Job drawing, mm, ordinate dimensions from the low corner. One solid piece. A direction names the side the tool comes from. Give positions to 0.01 mm unless a question says otherwise; leave off trailing zeros. Order: outer loops, then holes, each group sorted by start corner. A loop starts at its lowest first (then second) coordinate and runs counter-clockwise, first axis right, second up. Notation, with made-up numbers: M 52,7 L 86,7 A14 cw 86,33 Z; hole C 24,-38.5 d1. An arc over 180 degrees is marked long. Use CSV: the item, a comma, the result in double quotes. Start each with the question number.
Item 1: Pin check, flat tips, straight feed: P1, Ø23, axis at x = 42, y = 43.5, coming from the +Z side; P2, Ø7.5, axis at x = 54, y = 95, coming from the +Z side; P3, Ø12.5, axis at x = 50.5, z = 11.5, coming from the -Y side. Stop position of each tip, or through.
Item 2: Band-saw the part on C-C on x = 80.5. Write the cut outline in (y, z).
Item 3: Which spindle directions (+Z, -Z, +X, -X, +Y, -Y) get a long thin tool onto all of the face, cutting with end or side? Do the marked faces 5, 6, 7 and 8. Say none if no direction does.
Item 4: Two-plate mould, pull along X, no slides. Class the marked faces 1, 2, 3 and 4: pulls with the +X half, pulls with the -X half, needs draft (parallel to the pull), parting line crosses it, or undercut.
Item 5: Band-saw the part on A-A on y = 12.5. Write the cut outline in (x, z), plus the area to 3 significant figures.
Item 6: Band-saw the part on D-D on z = 13. Write the cut outline in (x, y), plus the area to 3 significant figures.
Item 7: Band-saw the part on B-B on z = 62. Write the cut outline in (x, y).
Item 8: Wall check: line 1 along X through (y, z) = (93, 73); line 2 along Z through (x, y) = (4, 30); line 3 along Y through (x, z) = (86, 84.5). Give the ranges that are in metal, low to high.
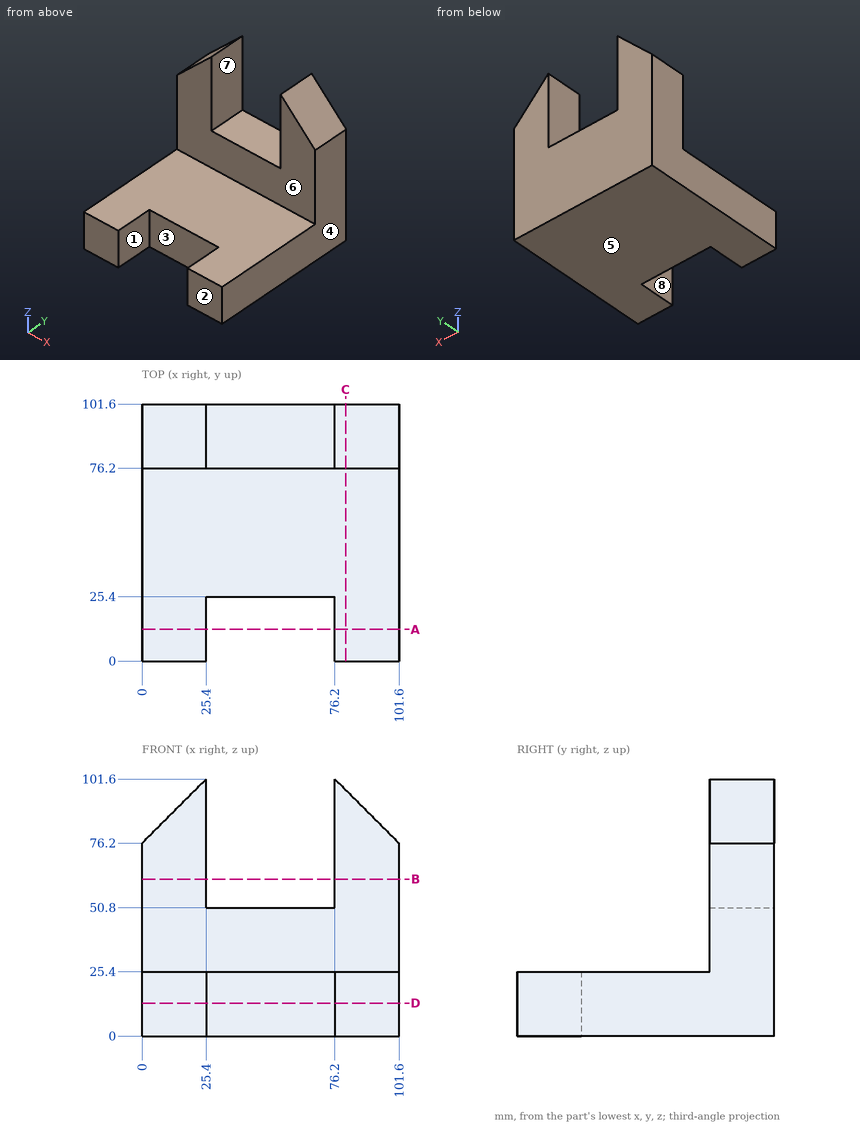
Model answer:
1,P1,"stops at z = 25.4"
1,P2,"stops at z = 50.8"
1,P3,"stops at y = 25.4"
2,outline,"M 0,0 L 101.6,0 L 101.6,97.3 L 76.2,97.3 L 76.2,25.4 L 0,25.4 Z"
3,face 5,"-Z, +X, -X, +Y, -Y"
3,face 6,"+Z, +X, -X, -Y"
3,face 7,"+Z, +Y, -Y"
3,face 8,"+Z, -Z, -Y"
4,face 1,"undercut"
4,face 2,"needs draft"
4,face 3,"undercut"
4,face 4,"pulls with the +X half"
5,outline,"M 0,0 L 25.4,0 L 25.4,25.4 L 0,25.4 Z; M 76.2,0 L 101.6,0 L 101.6,25.4 L 76.2,25.4 Z"
5,area,"1,290 mm^2"
6,outline,"M 0,0 L 25.4,0 L 25.4,25.4 L 76.2,25.4 L 76.2,0 L 101.6,0 L 101.6,101.6 L 0,101.6 Z"
6,area,"9,030 mm^2"
7,outline,"M 0,76.2 L 25.4,76.2 L 25.4,101.6 L 0,101.6 Z; M 76.2,76.2 L 101.6,76.2 L 101.6,101.6 L 76.2,101.6 Z"
8,line 1,"x = 0 to 25.4, 76.2 to 101.6"
8,line 2,"z = 0 to 25.4"
8,line 3,"y = 76.2 to 101.6"
